Here's how the part is built. I have some questions about the finished solid (model axes, mm). A direction names the side the tool comes from. Give positions to 0.01 mm unless a question says otherwise; leave off trailing zeros. Loops run counter-clockwise (first coordinate to the right, second up) from the corner with the lowest first, then second, coordinate; pieces in that order, holes last. Notation, with made-up numbers: M -33.75,-26 L -3.75,-26 A18 cw -3.75,-14 Z; hole C -4.75,15.25 d4. An arc over 180 degrees is marked long. Write item = value, one per line. Start each with the question number.
Autodesk Inventor part; units mm, degrees
ref_plane "ANBAU_XY" through (0, 0, 0) normal (0, 0, 1) x (1, 0, 0)
ref_plane "ANBAU_YZ" through (0, 0, 0) normal (1, 0, 0) x (0, 1, 0)
ref_plane "ANBAU_ZX" through (0, 0, 0) normal (0, 1, 0) x (0, 0, 1)
sketch "Sketch_1" plane through (0, 0, 0) normal (1, 0, 0) x (0, 1, 0)
  line L0 (0, -48.4) -> (0, 0)
  line L1 (0, 0) -> (5, 0)
  line L2 (5, 0) -> (5, -33.94)
  line L3 (5, -33.94) -> (4.54, -34.4)
  line L4 (4.54, -34.4) -> (4, -34.4)
  line L5 (4, -34.4) -> (4, -47.9)
  line L6 (4, -47.9) -> (3.5, -48.4)
  line L7 (3.5, -48.4) -> (0, -48.4)
  line L8 (0, -48.4) -> (0, 0)
revolve "Revolution1" add sketch "Sketch_1" angle 360 about axis through (0, 0, -48.4) along (0, 0, -1)
thread "Thread1"
ref_plane "ANBAU_XY" through (0, 0, 0) normal (0, 0, 1) x (1, 0, 0)
ref_plane "ANBAU_YZ" through (0, 0, 0) normal (1, 0, 0) x (0, 1, 0)
ref_plane "ANBAU_ZX" through (0, 0, 0) normal (0, 1, 0) x (0, 0, 1)
properties part number "ESBF-BS-40-ESBF-BS-40---(KSA)"
Q1. If we section it at A-A, the plane x = 0: List the corners of the cut face in (y, z) for me, then the cut area to 3 significant figures.
Q2. Will these pins go through, and if not, where does the flat tip stop? pin 1 (4 mm diameter, centred on x = 4, z = -40.5, fed in from -Y); pin 2 (1.5 mm diameter, centred on y = -3, z = -37.5, fed in from -X); pin 3 (4 mm diameter, centred on y = -3, z = -43.5, fed in from +X).
Q3. If I drill on line 1 along X through (y, z) = (0.25, -44.5); line 2 along X through (y, z) = (0.25, -13); line 3 along Z through (x, y) = (-0.75, -4), over which ranges is the centre line in solid material (lowest first)?
Q4. On a 3-axis mill with a long thin cutter (end or side, diameter ignored), from which of +Z, -Z, +X, -X, +Y, -Y can I reach the whole of each face in a straight line? I mean faces 1 (the flat face through (0, 0, 0)), 2 (the flat face through (-3, 3, -34.4)). Say none if no direction works.
Q5. If we section it at C-C, the plane z = -4.5: List the corners of the cut face in (x, y) for me, then the cut area to 3 significant figures.
Q6. If we section it at D-D, the plane z = -39.5: List the corners of the cut face in (x, y) for me.
Resolved:
q1.outline = M -5,-33.94 L -4.54,-34.4 L -4,-34.4 L -4,-47.9 L -3.5,-48.4 L 3.5,-48.4 L 4,-47.9 L 4,-34.4 L 4.54,-34.4 L 5,-33.94 L 5,0 L -5,0 Z
q1.area = 456 mm²
q2.pin_1 = -3.46
q2.pin_2 = -3.31
q2.pin_3 = 3.87
q3.line_1 = -3.99 to 3.99
q3.line_2 = -4.99 to 4.99
q3.line_3 = -34.4 to 0
q4.face_1 = +Z, +X, -X, +Y, -Y
q4.face_2 = -Z
q5.outline = C 0,0 d10
q5.area = 78.5 mm²
q6.outline = C 0,0 d8
